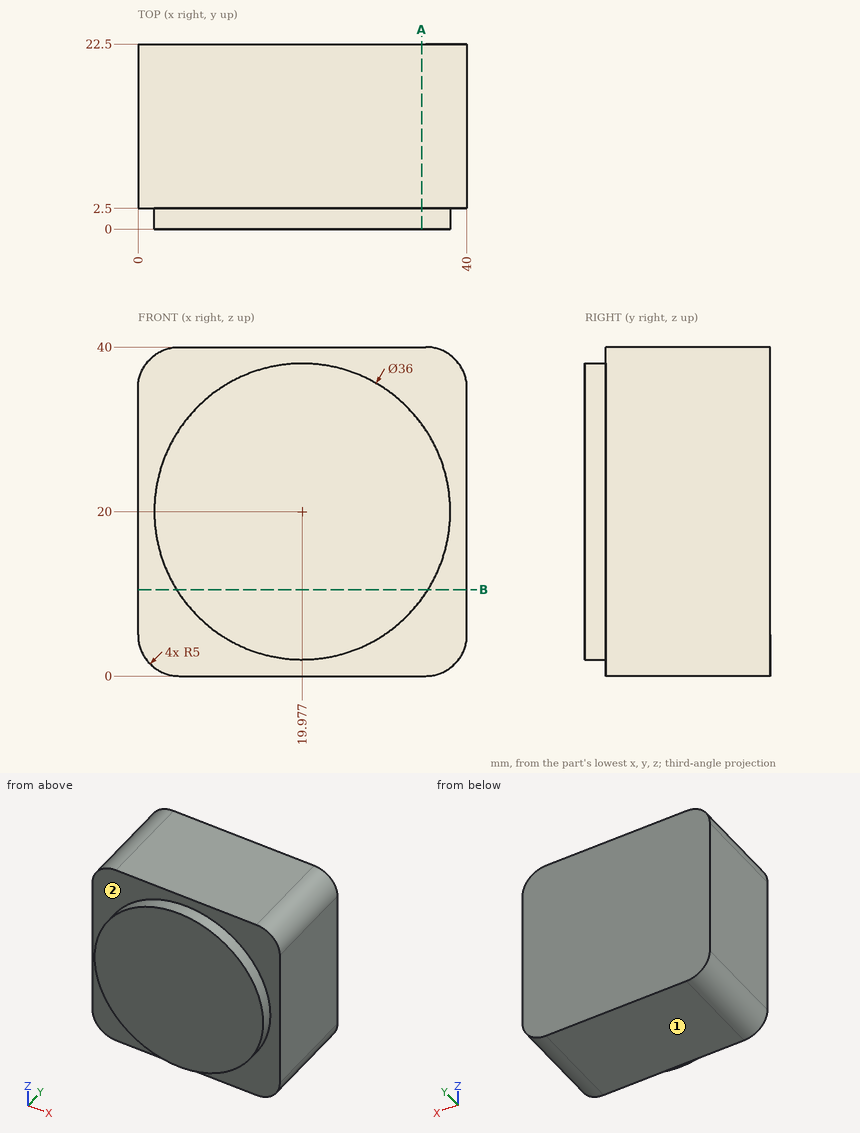
Input: dimensioned drawing with shaded views. Units: mm. Origin: part minimum x, y, z. A direction names the side the tool comes from. Round coordinates to 2 decimals unless told otherwise and drop trailing zeros. Loops run counter-clockwise (first coordinate to the right, second up) from the corner with the lowest first, then second, coordinate; pieces in that order, holes last. Notation, with made-up numbers: (18, 40) -> (36, 40) arc R29 cw to (36, 62) -> close; hole circle Ø3 at (22.25, -11). An arc over 180 degrees is marked (long way). Answer as a JSON object with one key per item and string values. Group by question number.
1) Pin query (flat end, axial travel): pin 1 (2 mm diameter, centred on x = 10.5, z = 14, fed in from -Y). Return the tip coordinate at first contact, or that it passes through.
2) Reachability of the marked faces 1 and 2 from +Z, -Z, +X, -X, +Y, -Y: full face, straight path, thin tool, end or side. Return the list, or none.
3) Section query A-A on x = 34.5. Output: boundary loops of the cut face in (y, z) (1 decimal), plus the area to 3 significant figures.
4) Ray query, L1, parallel to Y at x = 4, z = 32; L2, parallel to X at y = 1.5, z = 21.5 (1 decimal); L3, parallel to Z at x = 4.5, y = 18.5 (1 decimal). Return the intervals inside material, ascending.
5) Section query B-B on z = 10.5. Output: boundary loops of the cut face in (x, y).
Reply:
{
 "1": {"pin 1": "stops at y = 0"},
 "2": {"face 1": "-Z, +X, -X, +Y, -Y", "face 2": "-Y"},
 "3": {"outline": "(0, 9.4) -> (2.5, 9.4) -> (2.5, 0) -> (22.5, 0) -> (22.5, 40) -> (2.5, 40) -> (2.5, 30.6) -> (0, 30.6) -> close", "area": "853 mm2"},
 "4": {"L1": "y = 2.5 to 22.5", "L2": "x = 2 to 37.9", "L3": "z = 0 to 40"},
 "5": {"outline": "(0, 2.5) -> (4.69, 2.5) -> (4.69, 0) -> (35.27, 0) -> (35.27, 2.5) -> (40, 2.5) -> (40, 22.5) -> (0, 22.5) -> close"}
}
